Geometry: see drawing. Coordinates: mm, zero at the bounding-box minimum. Give positions to 0.01 mm unless a question says otherwise; leave off trailing zeros. Use a Markdown table: item, result.
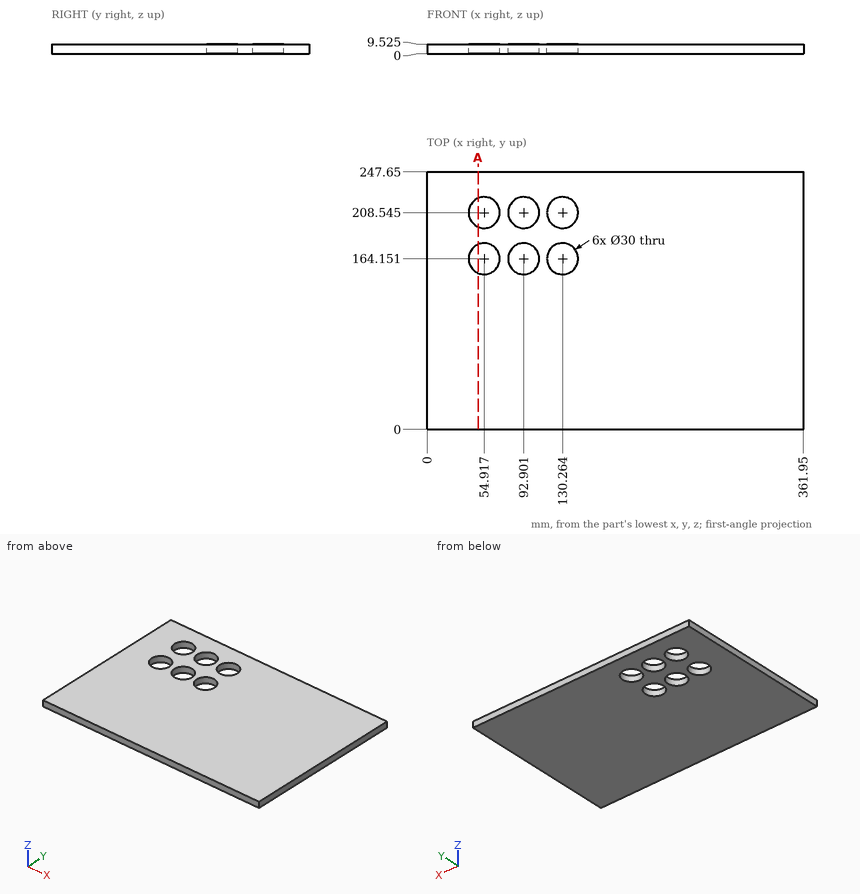
1) First-contact query: pin 1 Ø24 at (x, y) = (92.9, 208.54) entering from -Z. Flat tip, straight axial feed; report the tip coordinate or a pass-through.
Response values:
| item | result |
|---|---|
| pin 1 | passes through |
2) Cut plane A-A on x = 49. State how many separate pieces and enclosed holes the cut face has, and give its area (3 significant figures).
Response values:
| item | result |
|---|---|
| separate pieces | 3 |
| enclosed holes | 0 |
| area | 1,830 mm² |
3) Material intervals for line 1 (Y direction, x = 92, z = 8.75); line 2 (Y direction, x = 136.5, z = 6.75), sorted ascending. Write a range as from..to.
Response values:
| item | result |
|---|---|
| line 1 | y = 0..149.18, 179.12..193.57, 223.52..247.65 |
| line 2 | y = 0..150.51, 177.79..194.9, 222.19..247.65 |
